```python
from build123d import *

# Parameters (mm, degrees)
SKETCH_1_W          = 30
SKETCH_1_H          = 30
EXTRUDE_1_DEPTH     = 30
CUT_EXTRUDE_1_DEPTH = 52.961524227
SKETCH_3_W          = 20
SKETCH_3_H          = 10
CUT_EXTRUDE_2_DEPTH = 52.961524227
SKETCH_4_W          = 10
SKETCH_4_H          = 10
CUT_EXTRUDE_3_DEPTH = 52.961524227


with BuildPart() as part:
    # 草圖1 → 填料-伸長1 (new body)
    with BuildSketch(Plane.XY):
        with Locations((15, 15)):
            Rectangle(SKETCH_1_W, SKETCH_1_H)
    extrude(amount=-EXTRUDE_1_DEPTH)

    # 草圖2 → 除料-伸長1 (cut, through all)
    with BuildSketch(Plane.XY):
        Polygon((30, 30), (10, 30), (10, 20), (20, 20), (20, 10), (30, 10), align=None)
    extrude(amount=-CUT_EXTRUDE_1_DEPTH, mode=Mode.SUBTRACT)

    # 草圖3 → 除料-伸長2 (cut, through all)
    with BuildSketch(Plane(origin=(0, 30, 0), x_dir=(1, 0, 0), z_dir=(0, 1, 0))):
        with Locations((20, 5)):
            Rectangle(SKETCH_3_W, SKETCH_3_H)
    extrude(amount=-CUT_EXTRUDE_2_DEPTH, mode=Mode.SUBTRACT)

    # 草圖4 → 除料-伸長3 (cut, through all)
    with BuildSketch(Plane(origin=(30, 0, 0), x_dir=(0, 0, -1), z_dir=(1, 0, 0))):
        with Locations((5, 25)):
            Rectangle(SKETCH_4_W, SKETCH_4_H)
    extrude(amount=-CUT_EXTRUDE_3_DEPTH, mode=Mode.SUBTRACT)


solid = part.part
```
Work out the finished part from the listing and answer in its coordinate system (mm). A direction names the side the tool comes from. Round coordinates to 2 decimals unless told otherwise and drop trailing zeros. Write each loop counter-clockwise with the first axis right and the second up, starting at its lowest first coordinate (ties: lowest second). Pieces come first, ordered by that corner, then holes.
1) Which of the six approach directions +Z, -Z, +X, -X, +Y, -Y give full straight-line access (tool end or side, diameter ignored) to faces 1 (the face through (18, 8, -10)), 2 (the face through (5, 25, -10)), 3 (the face through (25, 10, -20)), 4 (the face through (11, 12, -30))?
2) A cutting plane is placed at A-A on z = -18.5. Determine the outline of the cut face in (x, y).
3) A cutting plane is placed at C-C on x = 6.75. Determine the outline of the cut face in (y, z), and give its area (3 significant figures).
4) A cutting plane is placed at D-D on x = 23. Determine the outline of the cut face in (y, z), and give its area (3 significant figures).
5) A cutting plane is placed at B-B on y = 9.5. Determine the outline of the cut face in (x, z), and give its area (3 significant figures).
6) Flat-ended cylindrical pins translate along their axes: P1, Ø8, axis at y = 25, z = -20, coming from the +X side; P2, Ø5, axis at x = 9.5, z = -6.5, coming from the -Y side; P3, Ø3, axis at x = 3, y = 26.5, coming from the +Z side; P4, Ø5, axis at y = 13, z = -20, coming from the +X side. Find the tip coordinate at first contact, or state that the pin passes through.
7) Consider probe 1 along Z at (x, y) = (3.75, 26.25); probe 2 along Y at (x, z) = (20.5, -11.5); probe 3 along X at (y, z) = (17, -17.5). Determine where each line is inside the solid, lowest interval first.
Entries:
1. face 1: +Z, +X, +Y, -Y
1. face 2: +Z, +X, -X, +Y
1. face 3: +Z, -Z, +X, +Y
1. face 4: -Z, +X, -X, +Y, -Y
2. outline: (0, 0) - (30, 0) - (30, 10) - (20, 10) - (20, 20) - (10, 20) - (10, 30) - (0, 30) - close
3. outline: (0, -30) - (30, -30) - (30, -10) - (20, -10) - (20, 0) - (0, 0) - close
3. area: 800 mm2
4. outline: (0, -30) - (10, -30) - (10, -10) - (0, -10) - close
4. area: 200 mm2
5. outline: (0, -30) - (30, -30) - (30, -10) - (10, -10) - (10, 0) - (0, 0) - close
5. area: 700 mm2
6. P1: stops at x = 10
6. P2: stops at y = 0
6. P3: stops at z = -10
6. P4: stops at x = 20
7. probe 1: z = -30 to -10
7. probe 2: y = 0 to 10
7. probe 3: x = 0 to 20
